from build123d import *

# Parameters (mm, degrees)
CROQUIS1_W              = 42.3
CROQUIS1_H              = 42.3
CROQUIS1_R              = 1.85
CROQUIS1_R_2            = 12
SALIENTE_EXTRUIR1_DEPTH = 2
CHAFL_N1_SIZE           = 4.09
CROQUIS2_R              = 6
CORTAR_EXTRUIR1_DEPTH   = 60.854657296
CROQUIS4_R              = 3.5
CORTAR_EXTRUIR3_DEPTH   = 60.854657296


with BuildPart() as part:
    # Croquis1 → Saliente-Extruir1 (new body)
    with BuildSketch(Plane.XY):
        with Locations((21.15, 21.15)):
            Rectangle(CROQUIS1_W, CROQUIS1_H)
        with Locations((5.65, 36.65)):
            Circle(CROQUIS1_R, mode=Mode.SUBTRACT)
        with Locations((5.65, 5.65)):
            Circle(CROQUIS1_R, mode=Mode.SUBTRACT)
        with Locations(Location((36.65, 5.65, 0), (0, 0, 180))):
            Circle(CROQUIS1_R, mode=Mode.SUBTRACT)
        with Locations(Location((36.65, 36.65, 0), (0, 0, 180))):
            Circle(CROQUIS1_R, mode=Mode.SUBTRACT)
        with Locations((21.15, 21.15)):
            Circle(CROQUIS1_R_2, mode=Mode.SUBTRACT)
    extrude(amount=SALIENTE_EXTRUIR1_DEPTH)

    # Chaflán1
    chafl_n1_edges = [part.edges().sort_by_distance(p)[0] for p in [
        (0, 42.3, 1),
        (42.3, 42.3, 1),
        (42.3, 0, 1),
        (0, 0, 1),
    ]]
    chamfer(chafl_n1_edges, length=CHAFL_N1_SIZE)

    # Croquis2 → Cortar-Extruir1 (cut, through all)
    with BuildSketch(Plane(origin=(0, 0, 0), x_dir=(-1, 0, 0), z_dir=(0, 0, -1))):
        with Locations((-42.3, 21.15)):
            Circle(CROQUIS2_R)
    extrude(amount=-CORTAR_EXTRUIR1_DEPTH, mode=Mode.SUBTRACT)

    # Croquis4 → Cortar-Extruir3 (cut, through all)
    with BuildSketch(Plane(origin=(0, 0, 0), x_dir=(-1, 0, 0), z_dir=(0, 0, -1))):
        with Locations((-5.65, 5.65)):
            Circle(CROQUIS4_R)
    extrude(amount=-CORTAR_EXTRUIR3_DEPTH, mode=Mode.SUBTRACT)


solid = part.part
Could you check a few things on this model? Use its own coordinates, in mm. Give positions to 0.01 mm unless a question says otherwise; leave off trailing zeros. Order: outer loops, then holes, each group sorted by start corner. A loop starts at its lowest first (then second) coordinate and runs counter-clockwise, first axis right, second up.
Item 1: I'm going to push a flat-ended pin straight in: pin 1 (3 mm diameter, centred on x = 5.65, y = 36.65, fed in from +Z). Where does the tip first touch, or does it pass through?
Item 2: If we section it at A-A, the plane y = 5.65: Write out the boundary of the cut face in (x, z), plus the area to 3 significant figures.
Item 3: I need wall thicknesses on line 1 (Y direction, x = 5.65, z = 0.5); line 2 (Y direction, x = 21.15, z = 1.1); line 3 (Y direction, x = 38, z = 1.5). Which ranges of each line are inside material? Lowest first, please.
Item 4: If we mould it in two halves opening along Y, with no side actions, what happens to faces 1 (the face through (5.409, 38.484, 0.986)), 2 (the face through (40.28, 2.07, 0.99)), 3 (the face through (42.3, 33, 1))? For each: pulls with the +Y half, pulls with the -Y half, needs draft (parallel to the pull), parting line crosses it, or undercut.
Item 5: If we section it at D-D, the plane x = 32.5: Write out the boundary of the cut face in (y, z), plus the area to 3 significant figures.
Item 6: If we section it at B-B, the plane y = 21.15: Write out the boundary of the cut face in (x, z).
Values:
1. pin 1: passes through
2. outline: (0, 0) - (2.15, 0) - (2.15, 2) - (0, 2) - close; (9.15, 0) - (34.8, 0) - (34.8, 2) - (9.15, 2) - close; (38.5, 0) - (42.3, 0) - (42.3, 2) - (38.5, 2) - close
2. area: 63.2 mm2
3. line 1: y = 0 to 2.15, 9.15 to 34.8, 38.5 to 42.3
3. line 2: y = 0 to 9.15, 33.15 to 42.3
3. line 3: y = 0 to 4.39, 6.91 to 16.97, 25.33 to 35.39, 37.91 to 42.3
4. face 1: undercut
4. face 2: pulls with the -Y half
4. face 3: needs draft
5. outline: (0, 0) - (17.25, 0) - (17.25, 2) - (0, 2) - close; (25.05, 0) - (42.3, 0) - (42.3, 2) - (25.05, 2) - close
5. area: 69.0 mm2
6. outline: (0, 0) - (9.15, 0) - (9.15, 2) - (0, 2) - close; (33.15, 0) - (36.3, 0) - (36.3, 2) - (33.15, 2) - close
